For this review, take the finished solid that the model builds, in its own axes (mm). Face numbers are marked on the shaded views. A direction names the side the tool comes from. Round coordinates to 2 decimals unless told otherwise and drop trailing zeros. Write each loop counter-clockwise with the first axis right and the second up, starting at its lowest first coordinate (ties: lowest second). Pieces come first, ordered by that corner, then holes. Notation, with made-up numbers: (32.25, -10.75) -> (85.25, -10.75) arc R34 cw to (85.25, 19.25) -> close; hole circle Ø8 at (-2, 6.25). An arc over 180 degrees is marked (long way). Answer in a Markdown table with one row per item.
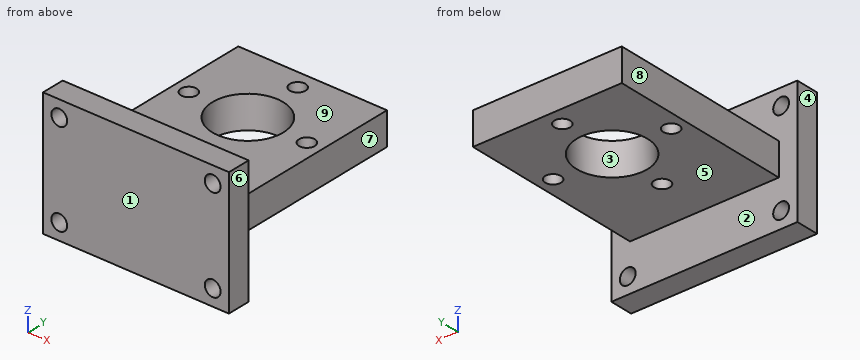
from build123d import *

# Parameters (mm, degrees)
SKETCH1_W           = 40
SKETCH1_H           = 27
SKETCH1_W_2         = 32
SKETCH1_H_2         = 7
BOSS_EXTRUDE1_DEPTH = 5
SKETCH1_3_W         = 32
SKETCH1_3_H         = 7
BOSS_EXTRUDE2_DEPTH = 45
CUT_EXTRUDE1_REACH  = 54.096
SKETCH2_R           = 7.62
CUT_EXTRUDE2_REACH  = 54.096
SKETCH4_R           = 1.7
CUT_EXTRUDE3_REACH  = 48.715
SKETCH5_R           = 1.7


with BuildPart() as part:
    # Sketch1 → Boss-Extrude1 (new body)
    with BuildSketch(Plane(origin=(0, 0, 0), x_dir=(1, 0, 0), z_dir=(0, 1, 0))):
        Rectangle(SKETCH1_W, SKETCH1_H)
        Rectangle(SKETCH1_W_2, SKETCH1_H_2, mode=Mode.SUBTRACT)
    extrude(amount=BOSS_EXTRUDE1_DEPTH)

    # Sketch1_3 → Boss-Extrude2 (add)
    with BuildSketch(Plane(origin=(0, 0, 0), x_dir=(1, 0, 0), z_dir=(0, 1, 0))):
        Rectangle(SKETCH1_3_W, SKETCH1_3_H)
    extrude(amount=BOSS_EXTRUDE2_DEPTH)

    # Sketch2 → Cut-Extrude1 (cut, up to next)
    with BuildSketch(Plane.XY.offset(3.5), mode=Mode.PRIVATE) as cut_extrude1_sk1:
        with Locations((0, 28.5)):
            Circle(SKETCH2_R)
    cut_extrude1_tool1 = extrude(cut_extrude1_sk1.sketch, amount=-CUT_EXTRUDE1_REACH, mode=Mode.PRIVATE) & part.part
    add(cut_extrude1_tool1.solids().sort_by_distance((0, 28.5, 3.5))[0], mode=Mode.SUBTRACT)

    # Sketch4 → Cut-Extrude2 (cut, up to next)
    with BuildSketch(Plane.XY.offset(3.5), mode=Mode.PRIVATE) as cut_extrude2_sk1:
        with Locations((0, 41.2)):
            Circle(SKETCH4_R)
    cut_extrude2_tool1 = extrude(cut_extrude2_sk1.sketch, amount=-CUT_EXTRUDE2_REACH, mode=Mode.PRIVATE) & part.part
    # Sketch4 → Cut-Extrude2 (cut, up to next)
    with BuildSketch(Plane.XY.offset(3.5), mode=Mode.PRIVATE) as cut_extrude2_sk2:
        with Locations((12.7, 28.5)):
            Circle(SKETCH4_R)
    cut_extrude2_tool2 = extrude(cut_extrude2_sk2.sketch, amount=-CUT_EXTRUDE2_REACH, mode=Mode.PRIVATE) & part.part
    # Sketch4 → Cut-Extrude2 (cut, up to next)
    with BuildSketch(Plane.XY.offset(3.5), mode=Mode.PRIVATE) as cut_extrude2_sk3:
        with Locations((0, 15.8)):
            Circle(SKETCH4_R)
    cut_extrude2_tool3 = extrude(cut_extrude2_sk3.sketch, amount=-CUT_EXTRUDE2_REACH, mode=Mode.PRIVATE) & part.part
    # Sketch4 → Cut-Extrude2 (cut, up to next)
    with BuildSketch(Plane.XY.offset(3.5), mode=Mode.PRIVATE) as cut_extrude2_sk4:
        with Locations((-12.7, 28.5)):
            Circle(SKETCH4_R)
    cut_extrude2_tool4 = extrude(cut_extrude2_sk4.sketch, amount=-CUT_EXTRUDE2_REACH, mode=Mode.PRIVATE) & part.part
    add(cut_extrude2_tool1.solids().sort_by_distance((0, 41.2, 3.5))[0], mode=Mode.SUBTRACT)
    add(cut_extrude2_tool2.solids().sort_by_distance((12.7, 28.5, 3.5))[0], mode=Mode.SUBTRACT)
    add(cut_extrude2_tool3.solids().sort_by_distance((0, 15.8, 3.5))[0], mode=Mode.SUBTRACT)
    add(cut_extrude2_tool4.solids().sort_by_distance((-12.7, 28.5, 3.5))[0], mode=Mode.SUBTRACT)

    # Sketch5 → Cut-Extrude3 (cut, up to next)
    with BuildSketch(Plane(origin=(0, 5, 0), x_dir=(1, 0, 0), z_dir=(0, 1, 0)), mode=Mode.PRIVATE) as cut_extrude3_sk1:
        with Locations(Location((-16.5, 10, 0), (0, 0, 270))):
            Circle(SKETCH5_R)
    cut_extrude3_tool1 = extrude(cut_extrude3_sk1.sketch, amount=-CUT_EXTRUDE3_REACH, mode=Mode.PRIVATE) & part.part
    # Sketch5 → Cut-Extrude3 (cut, up to next)
    with BuildSketch(Plane(origin=(0, 5, 0), x_dir=(1, 0, 0), z_dir=(0, 1, 0)), mode=Mode.PRIVATE) as cut_extrude3_sk2:
        with Locations(Location((-16.5, -10, 0), (0, 0, 270))):
            Circle(SKETCH5_R)
    cut_extrude3_tool2 = extrude(cut_extrude3_sk2.sketch, amount=-CUT_EXTRUDE3_REACH, mode=Mode.PRIVATE) & part.part
    # Sketch5 → Cut-Extrude3 (cut, up to next)
    with BuildSketch(Plane(origin=(0, 5, 0), x_dir=(1, 0, 0), z_dir=(0, 1, 0)), mode=Mode.PRIVATE) as cut_extrude3_sk3:
        with Locations(Location((16.5, -10, 0), (0, 0, 90))):
            Circle(SKETCH5_R)
    cut_extrude3_tool3 = extrude(cut_extrude3_sk3.sketch, amount=-CUT_EXTRUDE3_REACH, mode=Mode.PRIVATE) & part.part
    # Sketch5 → Cut-Extrude3 (cut, up to next)
    with BuildSketch(Plane(origin=(0, 5, 0), x_dir=(1, 0, 0), z_dir=(0, 1, 0)), mode=Mode.PRIVATE) as cut_extrude3_sk4:
        with Locations(Location((16.5, 10, 0), (0, 0, 90))):
            Circle(SKETCH5_R)
    cut_extrude3_tool4 = extrude(cut_extrude3_sk4.sketch, amount=-CUT_EXTRUDE3_REACH, mode=Mode.PRIVATE) & part.part
    add(cut_extrude3_tool1.solids().sort_by_distance((-16.5, 5, -10))[0], mode=Mode.SUBTRACT)
    add(cut_extrude3_tool2.solids().sort_by_distance((-16.5, 5, 10))[0], mode=Mode.SUBTRACT)
    add(cut_extrude3_tool3.solids().sort_by_distance((16.5, 5, 10))[0], mode=Mode.SUBTRACT)
    add(cut_extrude3_tool4.solids().sort_by_distance((16.5, 5, -10))[0], mode=Mode.SUBTRACT)


solid = part.part
1) For the marked faces 5, 6, 7, 8 and 9, list the 3-axis set-ups (+Z, -Z, +X, -X, +Y, -Y) from which the entire face can be reached by the end or side of a thin tool; tool diameter is ignored.
Solved:
| item | result |
|---|---|
| face 5 | -Z, +X, -X, +Y |
| face 6 | +Z, -Z, +X, +Y, -Y |
| face 7 | +Z, -Z, +X, +Y |
| face 8 | +Z, -Z, -X, +Y |
| face 9 | +Z, +X, -X, +Y |
2) Consider section A-A on x = -12.7. State the section outline as (y, z) points, then the cut area to 3 significant figures.
Solved:
| item | result |
|---|---|
| outline | (0, -13.5) -> (5, -13.5) -> (5, -3.5) -> (26.8, -3.5) -> (26.8, 3.5) -> (5, 3.5) -> (5, 13.5) -> (0, 13.5) -> close; (30.2, -3.5) -> (45, -3.5) -> (45, 3.5) -> (30.2, 3.5) -> close |
| area | 391 mm² |
3) Consider section B-B on y = 15.8. State the section outline as (x, z) points, then the cut area to 3 significant figures.
Solved:
| item | result |
|---|---|
| outline | (-16, -3.5) -> (-1.7, -3.5) -> (-1.7, 3.5) -> (-16, 3.5) -> close; (1.7, -3.5) -> (16, -3.5) -> (16, 3.5) -> (1.7, 3.5) -> close |
| area | 200 mm² |
4) Mouldability with a two-part tool opening along Y and no side actions: class the marked faces 1, 2, 3 and 4 as pulls with the +Y half, pulls with the -Y half, needs draft (parallel to the pull), parting line crosses it, or undercut.
Solved:
| item | result |
|---|---|
| face 1 | pulls with the -Y half |
| face 2 | pulls with the +Y half |
| face 3 | undercut |
| face 4 | needs draft |
5) For line 1 (X direction, y = 3.1, z = 10); line 2 (Y direction, x = -12.7, z = -1.25); line 3 (Z direction, x = 12.5, y = 6.5), list the stretches that pass through material, from the lowest coordinate up. Write a range as [from, to].
Solved:
| item | result |
|---|---|
| line 1 | [-20, -18.2], [-14.8, 14.8], [18.2, 20] |
| line 2 | [0, 26.8], [30.2, 45] |
| line 3 | [-3.5, 3.5] |
6) Clearance check with flat-ended pins moving along their axes: pin 1 Ø10 at (y, z) = (19, 6) entering from +X; pin 2 Ø4.5 at (x, z) = (16.5, 10) entering from +Y; pin 3 Ø3 at (x, y) = (-1.5, 12) entering from +Z. State where each tip first meets the part, or that it passes through.
Solved:
| item | result |
|---|---|
| pin 1 | x = 16 |
| pin 2 | y = 5 |
| pin 3 | z = 3.5 |
7) Consider section D-D on x = 0. State the section outline as (y, z) points.
Solved:
| item | result |
|---|---|
| outline | (0, -13.5) -> (5, -13.5) -> (5, -3.5) -> (14.1, -3.5) -> (14.1, 3.5) -> (5, 3.5) -> (5, 13.5) -> (0, 13.5) -> close; (17.5, -3.5) -> (20.88, -3.5) -> (20.88, 3.5) -> (17.5, 3.5) -> close; (36.12, -3.5) -> (39.5, -3.5) -> (39.5, 3.5) -> (36.12, 3.5) -> close; (42.9, -3.5) -> (45, -3.5) -> (45, 3.5) -> (42.9, 3.5) -> close |
8) Consider section C-C on z = -10. State the section outline as (x, y) points, then the cut area to 3 significant figures.
Solved:
| item | result |
|---|---|
| outline | (-20, 0) -> (-18.2, 0) -> (-18.2, 5) -> (-20, 5) -> close; (-14.8, 0) -> (14.8, 0) -> (14.8, 5) -> (-14.8, 5) -> close; (18.2, 0) -> (20, 0) -> (20, 5) -> (18.2, 5) -> close |
| area | 166 mm² |
